from build123d import *

# Parameters (mm, degrees)
SKETCH_1_W               = 175
SKETCH_1_H               = 10
EXTRUDE_1_DEPTH          = 2
CUT_EXTRUDE_1_DEPTH      = 12
CUT_EXTRUDE_1_DEPTH_BACK = 15
SKETCH_2_R               = 3
SKETCH_3_R               = 3
SKETCH_3_R_2             = 0.75
CUT_EXTRUDE_2_DEPTH      = 10
FILLET_1_R               = 2


with BuildPart() as part:
    # 草图1 → 凸台-拉伸1 (new body)
    with BuildSketch(Plane.XY):
        with Locations((-82.5, -5)):
            Rectangle(SKETCH_1_W, SKETCH_1_H)
    extrude(amount=EXTRUDE_1_DEPTH)

    # 草图2 → 切除-拉伸1 (cut, two sides: drawn at the far end of the back side and taken through both)
    with BuildSketch(Plane.XY.offset(2).offset(-CUT_EXTRUDE_1_DEPTH_BACK)):
        with Locations((-162, -5)):
            Circle(SKETCH_2_R)
    extrude(amount=CUT_EXTRUDE_1_DEPTH + CUT_EXTRUDE_1_DEPTH_BACK, mode=Mode.SUBTRACT)

    # 草图3 → 切除-拉伸2 (cut)
    with BuildSketch(Plane.XY.offset(2)):
        with Locations((-3, -5)):
            Circle(SKETCH_3_R)
        with Locations((-8, -5)):
            Circle(SKETCH_3_R_2)
        with Locations((2, -5)):
            Circle(SKETCH_3_R_2)
    extrude(amount=-CUT_EXTRUDE_2_DEPTH, mode=Mode.SUBTRACT)

    # 圆角1
    fillet_1_edges = [part.edges().sort_by_distance(p)[0] for p in [
        (-170, 0, 1),
        (5, 0, 1),
        (5, -10, 1),
        (-170, -10, 1),
    ]]
    fillet(fillet_1_edges, radius=FILLET_1_R)


solid = part.part
The listing builds one solid part. Answer for the finished solid, in the listing's coordinates (mm). Give positions to 0.01 mm unless a question says otherwise; leave off trailing zeros. Loops run counter-clockwise (first coordinate to the right, second up) from the corner with the lowest first, then second, coordinate; pieces in that order, holes last. Notation, with made-up numbers: M -33.75,48 L 19.25,48 A14 ccw 19.25,70 Z; hole C 26.5,-28 d3. An arc over 180 degrees is marked long. Answer as CSV lines item,"result".
Item 1: The part is cut by section B-B (z = 1.7). Give the vertices of the cut face in (x, y), and give its area (3 significant figures).
Values follow:
outline,"M -170,-8 A2 ccw -168,-10 L 3,-10 A2 ccw 5,-8 L 5,-2 A2 ccw 3,0 L -168,0 A2 ccw -170,-2 Z; hole C -162,-5 d6; hole C -8,-5 d1.5; hole C -3,-5 d6; hole C 2,-5 d1.5"
area,"1,690 mm^2"
Item 2: Straight lines are drawn through the part: line 1 along X through (y, z) = (-3, 1.3); line 2 along X through (y, z) = (-7.25, 1.2); line 3 along X through (y, z) = (-4.5, 0.1). For each, find the intervals that lie inside material, in ascending order. Write a range as [from, to].
Values follow:
line 1,"x = [-170, -164.24], [-159.76, -5.24], [-0.76, 5]"
line 2,"x = [-170, -163.98], [-160.02, -4.98], [-1.02, 5]"
line 3,"x = [-170, -164.96], [-159.04, -8.56], [-7.44, -5.96], [-0.04, 1.44], [2.56, 5]"
Item 3: The part is cut by section A-A (x = -3). Give the vertices of the cut face in (y, z), and give its area (3 significant figures).
Values follow:
outline,"M -10,0 L -8,0 L -8,2 L -10,2 Z; M -2,0 L 0,0 L 0,2 L -2,2 Z"
area,"8.00 mm^2"
Item 4: The mould has two halves that part along Y. Classify faces 1 (the cylindrical face through (-3, -2, 1)), 2 (the flat face through (-84, -5, 0)): released by +Y, released by -Y, zero draft, split by the parting line, or undercut.
Values follow:
face 1,"undercut"
face 2,"zero draft"
